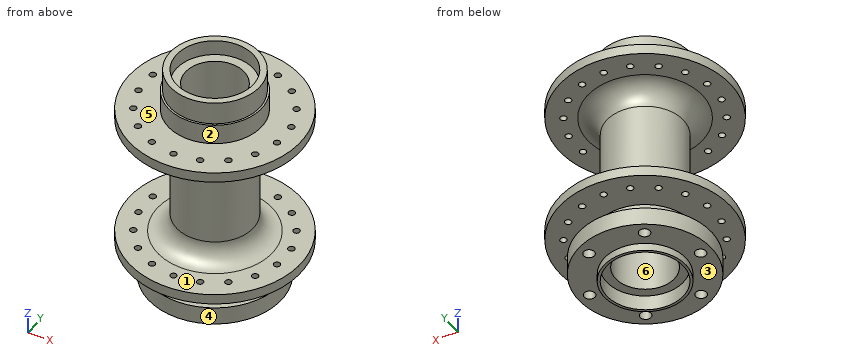
```python
from build123d import *

# Parameters (mm, degrees)
FILLET1_R                 = 7.5
FILLET2_R                 = 2.5
CUT_EXTRUDE1_DEPTH        = 67.034082109
CUT_EXTRUDE1_DEPTH_BACK   = 67.034082109
SKETCH3_R                 = 1.25
M5X0_8_TAPPED_HOLE1_D     = 4.2
M5X0_8_TAPPED_HOLE1_DEPTH = 7.000101775


with BuildPart() as part:
    # Sketch2 → Revolve1 (revolve)
    with BuildSketch(Plane(origin=(0, 0, 0), x_dir=(1, 0, 0), z_dir=(0, 1, 0)), mode=Mode.PRIVATE) as revolve1_sk:
        Polygon((15, 46), (16, 46), (16, 43), (26, 43), (26, 35.999898225), (18.25, 35.999898225), (18.25, 27.999898225), (33.5, 27.999898225), (33.5, 23.999898225), (15, 23.999898225), (15, -25.000101775), (33.5, -25.000101775), (33.5, -29.000101775), (18.25, -29.000101775), (18.25, -37.000101775), (17.5, -37.000101775), (17.5, -46), (15, -46), (15, -40), (11.5, -40), (11.5, 40), (15, 40), align=None)
    revolve(revolve1_sk.sketch.rotate(Axis((0, 0, -29.097498156), (0, 0, 1)), 180), axis=Axis((0, 0, -29.097498156), (0, 0, 1)))

    # Fillet1
    fillet1_edges = [part.edges().sort_by_distance(p)[0] for p in [
        (15, 0, 25.000101775),
        (15, 0, -23.999898225),
    ]]
    fillet(fillet1_edges, radius=FILLET1_R)

    # Fillet2
    fillet2_edges = [part.edges().sort_by_distance(p)[0] for p in [
        (18.25, 0, -35.999898225),
    ]]
    fillet(fillet2_edges, radius=FILLET2_R)

    # Sketch3 → Cut-Extrude1 (cut, two sides: drawn at the far end of the back side and taken through both)
    with BuildSketch(Plane.XY.offset(-CUT_EXTRUDE1_DEPTH_BACK)):
        with Locations((0, 27.25)):
            Circle(SKETCH3_R)
        with Locations((9.320048906, 25.606623916)):
            Circle(SKETCH3_R)
        with Locations((17.515962364, 20.874711075)):
            Circle(SKETCH3_R)
        with Locations((23.599192253, 13.625)):
            Circle(SKETCH3_R)
        with Locations((26.83601127, 4.731912841)):
            Circle(SKETCH3_R)
        with Locations((26.83601127, -4.731912841)):
            Circle(SKETCH3_R)
        with Locations((23.599192253, -13.625)):
            Circle(SKETCH3_R)
        with Locations((17.515962364, -20.874711075)):
            Circle(SKETCH3_R)
        with Locations((9.320048906, -25.606623916)):
            Circle(SKETCH3_R)
        with Locations((0, -27.25)):
            Circle(SKETCH3_R)
        with Locations((-9.320048906, -25.606623916)):
            Circle(SKETCH3_R)
        with Locations((-17.515962364, -20.874711075)):
            Circle(SKETCH3_R)
        with Locations((-23.599192253, -13.625)):
            Circle(SKETCH3_R)
        with Locations((-26.83601127, -4.731912841)):
            Circle(SKETCH3_R)
        with Locations((-26.83601127, 4.731912841)):
            Circle(SKETCH3_R)
        with Locations((-23.599192253, 13.625)):
            Circle(SKETCH3_R)
        with Locations((-17.515962364, 20.874711075)):
            Circle(SKETCH3_R)
        with Locations((-9.320048906, 25.606623916)):
            Circle(SKETCH3_R)
    extrude(amount=CUT_EXTRUDE1_DEPTH + CUT_EXTRUDE1_DEPTH_BACK, mode=Mode.SUBTRACT)

    # M5x0.8 Tapped Hole1
    with Locations(Plane(origin=(0, 0, -43), x_dir=(-1, 0, 0), z_dir=(0, 0, -1))):
        with Locations((-10.75, 18.619546181), (10.75, 18.619546181), (21.5, 0), (10.75, -18.619546181), (-10.75, -18.619546181), (-21.5, 0)):
            Hole(M5X0_8_TAPPED_HOLE1_D / 2, depth=M5X0_8_TAPPED_HOLE1_DEPTH)


solid = part.part
```
CAD build for the part. Positions are in the model's coordinates, mm. Face numbers are marked on the shaded views. A direction names the side the tool comes from. Coordinates: 2 decimals unless noted, no trailing zeros. Loops run counter-clockwise (first coordinate to the right, second up) from the corner with the lowest first, then second, coordinate; pieces in that order, holes last. Notation, with made-up numbers: (79, -19) - (131, -19) arc R18 cw to (131, 5) - close; hole circle Ø8 at (34.5, 36.5). An arc over 180 degrees is marked (long way). Return JSON: item names as keys, results as strings.
1. Band-saw the part on D-D (z = -4). Give the cut face in (x, y), and give its area (3 significant figures).
Result:
{"outline": "circle Ø30 at (0, 0); hole circle Ø23 at (0, 0)", "area": "291 mm2"}
2. Band-saw the part on B-B (x = 0). State how many separate pieces and enclosed holes the cut face has, and give its area (3 significant figures).
Result:
{"separate pieces": "6", "enclosed holes": "0", "area": "1,180 mm2"}
3. Probe L1, parallel to Z at x = -4, y = -23; L2, parallel to Z at x = 16.5, y = -27; L3, parallel to X at y = 5, z = 7. List the from-to ranges inside material, lowest first. Write a range as from..to.
Result:
{"L1": "z = -43..-36, -28..-24, 25..29", "L2": "z = -28..-24, 25..29", "L3": "x = -14.14..-10.36, 10.36..14.14"}
4. Band-saw the part on A-A (z = 32). Give the cut face in (x, y).
Result:
{"outline": "circle Ø36.5 at (0, 0); hole circle Ø23 at (0, 0)"}
5. 3-axis set-ups, long thin cutter, end or side, ignore diameter. For the marked faces 1, 2 and 3: which of +Z, -Z, +X, -X, +Y, -Y reach the whole face in a straight line?
Result:
{"face 1": "none", "face 2": "+Z", "face 3": "-Z"}
6. Mould opens along X. For the marked faces 4, 5 and 6 say: released by +X, released by -X, zero draft, split by the parting line, or undercut.
Result:
{"face 4": "split by the parting line", "face 5": "zero draft", "face 6": "undercut"}
7. Drop flat-ended pins along their axis: pin 1 (6 mm diameter, centred on x = -14.5, y = -26.5, fed in from -Z); pin 2 (3 mm diameter, centred on x = -22, z = 28.5, fed in from +Y); pin 3 (12 mm diameter, centred on x = 0, z = -18.5, fed in from +Y); pin 4 (1.5 mm diameter, centred on x = -26.84, y = -4.73, fed in from +Z). Give the stop position or say it passes through.
Result:
{"pin 1": "stops at z = -28", "pin 2": "stops at y = 26.5", "pin 3": "stops at y = 33.5", "pin 4": "passes through"}
